```python
from build123d import *

# Parameters (mm, degrees)
SKETCH_1_R                       = 42
SKETCH_1_R_2                     = 35.5
EXTRUDE_1_DEPTH                  = 25
SKETCH_2_R                       = 38
CUT_EXTRUDE_1_DEPTH              = 8
HOLE_WIZARD_M3_1_D               = 2.5
HOLE_WIZARD_M3_1_DEPTH           = 6
HOLE_WIZARD_M3_1_TIP             = 0.751075774
SKETCH_10_R                      = 44
SKETCH_10_R_2                    = 42
EXTRUDE_2_DEPTH                  = 6
CHAMFER_1_SIZE                   = 1
HOLE_WIZARD_M3_3_D               = 2.5
HOLE_WIZARD_M3_3_DEPTH           = 5
HOLE_WIZARD_M3_3_TIP             = 0.751075774
HOLE_WIZARD_M3_3_ON_FACE_2_D     = 2.5
HOLE_WIZARD_M3_3_ON_FACE_2_DEPTH = 5
HOLE_WIZARD_M3_3_ON_FACE_2_TIP   = 0.751075774
CHAMFER_2_SIZE                   = 1


with BuildPart() as part:
    # 草图1 → 凸台-拉伸1 (new body)
    with BuildSketch(Plane.XY):
        Circle(SKETCH_1_R)
        Circle(SKETCH_1_R_2, mode=Mode.SUBTRACT)
    extrude(amount=EXTRUDE_1_DEPTH)

    # 草图2 → 切除-拉伸1 (cut)
    with BuildSketch(Plane.XY.offset(25)):
        Circle(SKETCH_2_R)
    extrude(amount=-CUT_EXTRUDE_1_DEPTH, mode=Mode.SUBTRACT)

    # M3 螺纹孔1
    with Locations(Plane(origin=(-33.341978046, 19.25, 0), x_dir=(-1, 0, 0), z_dir=(0, 0, -1))):
        with Locations((0, 0), (0, -38.5), (-33.341978046, -57.75), (-66.683956092, -38.5), (-66.683956092, 0), (-33.341978046, 19.25)):
            Hole(HOLE_WIZARD_M3_1_D / 2, depth=HOLE_WIZARD_M3_1_DEPTH)
            with Locations((0, 0, -(HOLE_WIZARD_M3_1_DEPTH + HOLE_WIZARD_M3_1_TIP / 2))):  # 118° drill point
                Cone(0, HOLE_WIZARD_M3_1_D / 2, HOLE_WIZARD_M3_1_TIP, mode=Mode.SUBTRACT)

    # 草图10 → 凸台-拉伸2 (add)
    with BuildSketch(Plane.XY.offset(25)):
        Circle(SKETCH_10_R)
        Circle(SKETCH_10_R_2, mode=Mode.SUBTRACT)
    extrude(amount=-EXTRUDE_2_DEPTH)

    # 倒角1
    chamfer_1_edges = [part.edges().sort_by_distance(p)[0] for p in [
        (-42, 0, 0),
    ]]
    chamfer(chamfer_1_edges, length=CHAMFER_1_SIZE)

    # M3 螺纹孔3
    with Locations(Plane(origin=(35.507041555, 20.5, 25), x_dir=(1, 0, 0), z_dir=(0, 0, 1))):
        with Locations((0, 0), (0, -41), (-35.507041555, 20.5), (-35.507041555, -61.5), (-71.01408311, -41), (-71.01408311, 0)):
            Hole(HOLE_WIZARD_M3_3_D / 2, depth=HOLE_WIZARD_M3_3_DEPTH)
            with Locations((0, 0, -(HOLE_WIZARD_M3_3_DEPTH + HOLE_WIZARD_M3_3_TIP / 2))):  # 118° drill point
                Cone(0, HOLE_WIZARD_M3_3_D / 2, HOLE_WIZARD_M3_3_TIP, mode=Mode.SUBTRACT)

    # M3 螺纹孔3 on face 2
    with Locations(Plane(origin=(84.616598131, -20.470458883, 0), x_dir=(1, 0, 0), z_dir=(0, 0, 1))):
        with Locations((0, 0)):
            Hole(HOLE_WIZARD_M3_3_ON_FACE_2_D / 2, depth=HOLE_WIZARD_M3_3_ON_FACE_2_DEPTH)
            with Locations((0, 0, -(HOLE_WIZARD_M3_3_ON_FACE_2_DEPTH + HOLE_WIZARD_M3_3_ON_FACE_2_TIP / 2))):  # 118° drill point
                Cone(0, HOLE_WIZARD_M3_3_ON_FACE_2_D / 2, HOLE_WIZARD_M3_3_ON_FACE_2_TIP, mode=Mode.SUBTRACT)

    # 倒角2
    chamfer_2_edges = [part.edges().sort_by_distance(p)[0] for p in [
        (-44, 0, 19),
        (-44, 0, 25),
    ]]
    chamfer(chamfer_2_edges, length=CHAMFER_2_SIZE)


solid = part.part
```
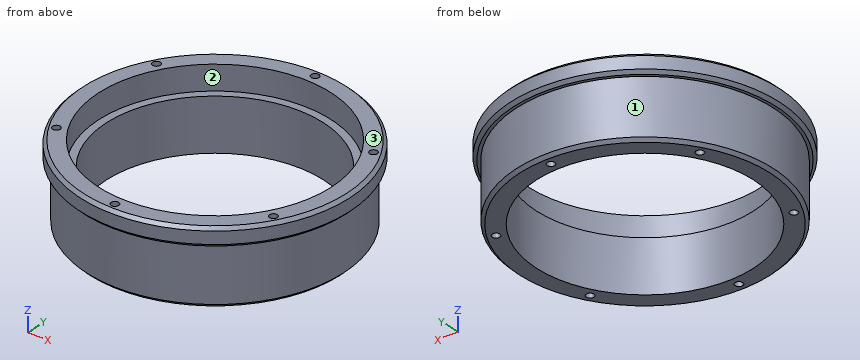
Geometry check sheet. Reference: the model listing, model coordinates, mm. Face numbers are marked on the shaded views. Coordinates: 2 decimals unless noted, no trailing zeros. Write each loop counter-clockwise with the first axis right and the second up, starting at its lowest first coordinate (ties: lowest second). Pieces come first, ordered by that corner, then holes. Notation, with made-up numbers: M 5,17 L 23,17 A37 ccw 23,54 Z; hole C 25,-25.75 d2. An arc over 180 degrees is marked long. Use one line per item in the form item = value. Start each with the question number.
1) Section check A-A on y = 0. Enter the section's corners in (x, z).
2) Section check B-B on z = 3.25. Enter the section's corners in (x, y), and give its area (3 significant figures).
3) Release check for a two-part mould opening along Y. For the marked faces 1, 2 and 3 record: pulls with the +Y half, pulls with the -Y half, needs draft (parallel to the pull), parting line crosses it, or undercut.
4) Thickness scan on probe 1 along Y at (x, z) = (0, 21.5); probe 2 along X at (y, z) = (-19.25, 4.75); probe 3 along X at (y, z) = (-20.5, 21.65). Record the ranges inside material, lowest first. Write a range as from..to.
5) Go/stop test with flat-tipped pins: pin 1 Ø10 at (x, z) = (-1.5, 19) entering from -Y; pin 2 Ø3 at (x, z) = (21.5, 14) entering from -Y; pin 3 Ø1.5 at (y, z) = (4.5, 9) entering from -X. Record where each tip stops, or that it passes through.
Responses:
q1.outline = M -44,20 L -43,19 L -42,19 L -42,1 L -41,0 L -35.5,0 L -35.5,17 L -38,17 L -38,25 L -43,25 L -44,24 Z; M 35.5,0 L 41,0 L 42,1 L 42,19 L 43,19 L 44,20 L 44,24 L 43,25 L 38,25 L 38,17 L 35.5,17 Z
q2.outline = C 0,0 d84; hole C 0,0 d71; hole C -33.34,-19.25 d2.5; hole C -33.34,19.25 d2.5; hole C 0,-38.5 d2.5; hole C 0,38.5 d2.5; hole C 33.34,-19.25 d2.5; hole C 33.34,19.25 d2.5
q2.area = 1,550 mm2
q3.face_1 = parting line crosses it
q3.face_2 = undercut
q3.face_3 = needs draft
q4.probe_1 = -44..-42.25, -39.75..-38, 38..39.75, 42.25..44
q4.probe_2 = -37.33..-34.59, -32.09..-29.83, 29.83..32.09, 34.59..37.33
q4.probe_3 = -38.93..-36.76, -34.26..-32, 32..34.26, 36.76..38.93
q5.pin_1 = -44
q5.pin_2 = -36.93
q5.pin_3 = -41.83
